The listing builds one solid part. Answer for the finished solid, in the listing's coordinates (mm). Coordinates: 2 decimals unless noted, no trailing zeros. Order: outer loops, then holes, each group sorted by start corner. A loop starts at its lowest first (then second) coordinate and runs counter-clockwise, first axis right, second up. Notation, with made-up numbers: (-19, -3.5) -> (19, -3.5) arc R26 ccw to (19, 12.5) -> close; hole circle Ø2 at (36, 26). An arc over 180 degrees is marked (long way). Answer in a Markdown table with one row per item.
```python
from build123d import *

# Parameters (mm, degrees)
ESQUISSE2_R             = 20
ENL_V_MAT_EXTRU_1_DEPTH = 58.940669043
TROU_TARAUD_M61_D       = 5
TROU_TARAUD_M61_DEPTH   = 17
TROU_TARAUD_M61_TIP     = 1.502151548
TROU_TARAUD_M62_D       = 5
TROU_TARAUD_M62_DEPTH   = 28
TROU_TARAUD_M62_TIP     = 1.502151548


with BuildPart() as part:
    # Esquisse1 → Révolution1 (revolve)
    with BuildSketch(Plane.XY, mode=Mode.PRIVATE) as r_volution1_sk:
        Polygon((0, 0), (40, 0), (40, 41.2), (30, 57.940669043), (0, 57.940669043), align=None)
    revolve(r_volution1_sk.sketch.rotate(Axis((0, 57.940669043, 0), (0, -1, 0)), 90), axis=Axis((0, 57.940669043, 0), (0, -1, 0)))  # turned: the seam where the file's is

    # Esquisse2 → Enlèv. mat.-Extru.1 (cut, through all)
    with BuildSketch(Plane(origin=(0, 57.940669043, 0), x_dir=(1, 0, 0), z_dir=(0, 1, 0))):
        with Locations(Location((0, 0, 0), (0, 0, 270))):  # turned: the seam where the file's is
            Circle(ESQUISSE2_R)
    extrude(amount=-ENL_V_MAT_EXTRU_1_DEPTH, mode=Mode.SUBTRACT)

    # Trou taraudé M61
    with Locations(Plane(origin=(-21.650635095, 57.940669043, -12.5), x_dir=(0, 0, 1), z_dir=(0, 1, 0))):
        with Locations((0, 0), (0, 43.30127019), (37.5, 21.650635095)):
            Hole(TROU_TARAUD_M61_D / 2, depth=TROU_TARAUD_M61_DEPTH)
            with Locations((0, 0, -(TROU_TARAUD_M61_DEPTH + TROU_TARAUD_M61_TIP / 2))):  # 118° drill point
                Cone(0, TROU_TARAUD_M61_D / 2, TROU_TARAUD_M61_TIP, mode=Mode.SUBTRACT)

    # Trou taraudé M62
    with Locations(Plane(origin=(0, 0, 30), x_dir=(0, 0, -1), z_dir=(0, -1, 0))):
        with Locations((0, 0), (30, 30), (60, 0), (30, -30)):
            Hole(TROU_TARAUD_M62_D / 2, depth=TROU_TARAUD_M62_DEPTH)
            with Locations((0, 0, -(TROU_TARAUD_M62_DEPTH + TROU_TARAUD_M62_TIP / 2))):  # 118° drill point
                Cone(0, TROU_TARAUD_M62_D / 2, TROU_TARAUD_M62_TIP, mode=Mode.SUBTRACT)


solid = part.part
```
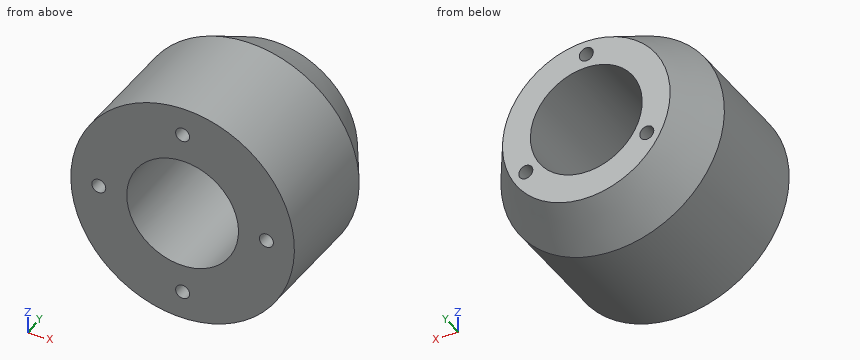
(1) Flat-ended cylindrical pins translate along their axes: pin 1 (2 mm diameter, centred on x = 14.5, y = 40.5, fed in from +Z); pin 2 (10 mm diameter, centred on y = 11.5, z = 24, fed in from -X); pin 3 (8 mm diameter, centred on x = 21.5, y = 45, fed in from +Z). Find the tip coordinate at first contact, or state that the pin passes through.
Check values:
| item | result |
|---|---|
| pin 1 | z = 37.65 |
| pin 2 | x = -35.2 |
| pin 3 | z = 34.74 |
(2) A cutting plane is placed at B-B, the plane y = 46. Determine the outline of the cut face in (x, z), then the cut area to 3 significant figures.
Check values:
| item | result |
|---|---|
| outline | circle Ø74.27 at (0, 0); hole circle Ø5 at (-21.65, -12.5); hole circle Ø40 at (0, 0); hole circle Ø5 at (0, 25); hole circle Ø5 at (21.65, -12.5) |
| area | 3,020 mm² |
(3) A cutting plane is placed at A-A, the plane y = 37. Determine the outline of the cut face in (x, z).
Check values:
| item | result |
|---|---|
| outline | circle Ø80 at (0, 0); hole circle Ø40 at (0, 0) |
(4) A cutting plane is placed at C-C, the plane y = 54.5. Determine the outline of the cut face in (x, z), then the cut area to 3 significant figures.
Check values:
| item | result |
|---|---|
| outline | circle Ø64.11 at (0, 0); hole circle Ø5 at (-21.65, -12.5); hole circle Ø40 at (0, 0); hole circle Ø5 at (0, 25); hole circle Ø5 at (21.65, -12.5) |
| area | 1,910 mm² |
(5) Find the intervals of material crossed by line 1 along X through (y, z) = (35.5, 0); line 2 along Z through (x, y) = (-0.5, 36.5); line 3 along X through (y, z) = (48.5, 25), in increasing order. Write a range as from..to.
Check values:
| item | result |
|---|---|
| line 1 | -40..-20, 20..40 |
| line 2 | -40..-19.99, 19.99..40 |
| line 3 | -25.4..-2.5, 2.5..25.4 |
